For this review, use the dimensioned drawing (mm, ordinates from the lowest corner) and the shaded views. Give positions to 0.01 mm unless a question says otherwise; leave off trailing zeros. Order: outer loops, then holes, each group sorted by start corner. A loop starts at its lowest first (then second) coordinate and runs counter-clockwise, first axis right, second up. Notation, with made-up numbers: M -14,-11 L 7,-11 A20 cw 7,12 Z; hole C -23,79 d1. An arc over 180 degrees is marked long. Use CSV: the item, a comma, the result in double quotes. Start each with the question number.
(1) Consider section B-B (x = 4.1). Write out the cut boundary in (y, z), and give its area (3 significant figures).
(2) Wall thickness on L1, parallel to X at y = 3.2, z = 41; L2, parallel to Y at x = 3.55, z = 17; L3, parallel to Y at x = 4.15, z = 39.5: over which ranges is each line inside the solid? List them lowest first. Write a range as from..to.
(3) Consider section A-A (z = 48). Write out the cut boundary in (x, y).
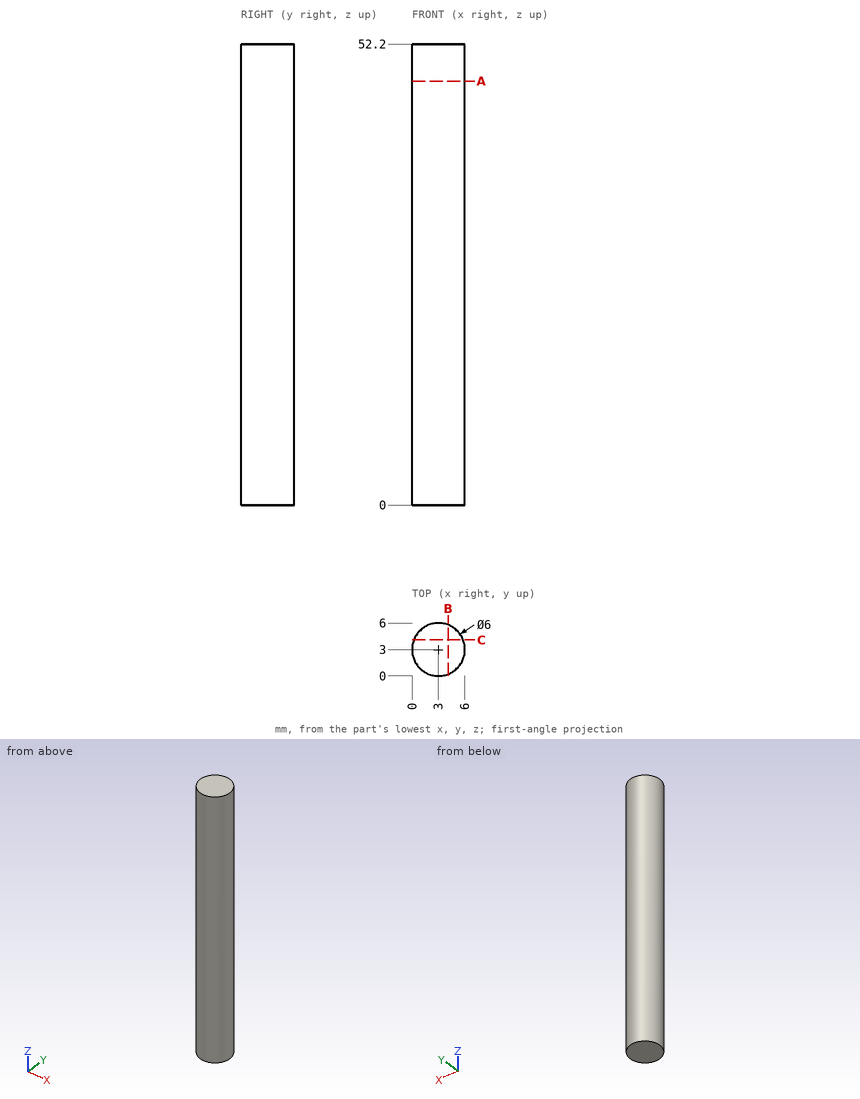
Check result:
1,outline,"M 0.21,0 L 5.79,0 L 5.79,52.2 L 0.21,52.2 Z"
1,area,"291 mm^2"
2,L1,"x = 0.01..5.99"
2,L2,"y = 0.05..5.95"
2,L3,"y = 0.23..5.77"
3,outline,"C 3,3 d6"
